```python
from build123d import *
from build123d import SkipClean  # not in build123d's __all__

# Parameters (mm, degrees)
F1_DEPTH = 31.75
F3_DEPTH = 12.7
F5_DEPTH = 12.7
F7_DEPTH = 25.401


with BuildPart() as f1:
    # F0 (on Top) → F1 (new body)
    with BuildSketch(Plane.XY):
        Polygon((31.597598396, 0), (0, -0.0003033445), (0, -38.1), (31.75, -38.1), (31.75, -25.4), (57.15, -25.4), (57.15, -12.7), (31.597598396, -12.7), align=None)
    extrude(amount=F1_DEPTH)

    # F2 (on face) → F3 (cut)
    with BuildSketch(Plane.XZ.offset(38.1)):
        Polygon((31.75, 0), (31.75, 31.75), (19.05, 31.75), align=None)
    extrude(amount=-F3_DEPTH, mode=Mode.SUBTRACT)

    # F4 (on face) → F5 (cut)
    with BuildSketch(Plane(origin=(2.9e-09, -0.0003033445, 0), x_dir=(-1, -9.6002e-06, 0), z_dir=(-9.6002e-06, 1, 0))):
        Polygon((-18.8975983945, 31.75), (-31.5975983945, 31.75), (-31.5975983945, 0), align=None)
    with SkipClean():  # cleaning this boolean's faces spoils the solid; the shape is the same uncleaned
        extrude(amount=-F5_DEPTH, mode=Mode.SUBTRACT)

    # F6 (on face) → F7 (cut, through all)
    with BuildSketch(Plane(origin=(0, -12.7, 0), x_dir=(-1, 0, 0), z_dir=(0, 1, 0))):
        Polygon((-44.373799198, 31.75), (-57.15, 31.75), (-57.15, 0), align=None)
    extrude(amount=-F7_DEPTH, mode=Mode.SUBTRACT)


solid = f1.part
```
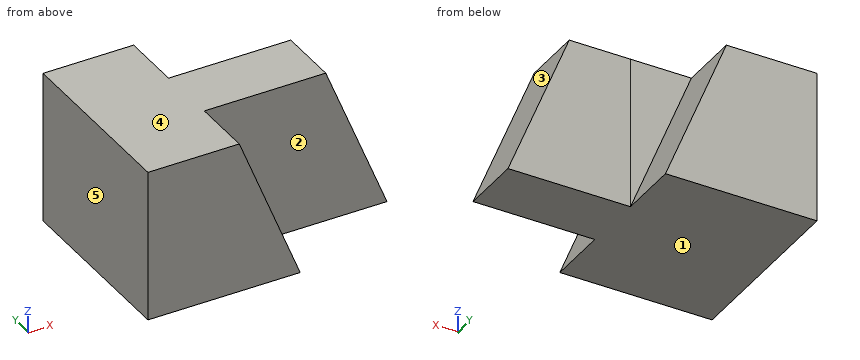
Design review of the part built by this model. Coordinates are the model's own, in mm. Face numbers are marked on the shaded views. A direction names the side the tool comes from. Give positions to 0.01 mm unless a question says otherwise; leave off trailing zeros. Order: outer loops, then holes, each group sorted by start corner. A loop starts at its lowest first (then second) coordinate and runs counter-clockwise, first axis right, second up. Notation, with made-up numbers: (44.25, -15) -> (85.25, -15) arc R26 ccw to (85.25, 4) -> close; hole circle Ø8 at (39, 61). An arc over 180 degrees is marked (long way). Write item = value, one per line. Start each with the question number.
(1) Mouldability with a two-part tool opening along X and no side actions: class the marked faces 3, 4 and 5 as +X half, -X half, draft (parallel to the pull), parting line (faces both ways), or undercut.
(2) We need section A-A on x = 23. Write out the cut boundary in (y, z) (3 decimals).
(3) For the marked faces 1 and 2, list the 3-axis set-ups (+Z, -Z, +X, -X, +Y, -Y) from which the entire face can be reached by the end or side of a thin tool; tool diameter is ignored.
(4) We need section D-D on z = 15. Write out the cut boundary in (x, y), plus the area to 3 significant figures.
(5) For pin 1 (2 mm diameter, centred on x = 19, y = -5, fed in from +Z); pin 2 (2 mm diameter, centred on x = 32, z = 9, fed in from -Y); pin 3 (1.5 mm diameter, centred on y = -4, z = 8, fed in from +X), all flat-tipped, find the tip position at first contact; note any pin that passes through.
(6) We need section B-B on z = 22. Write out the cut boundary in (x, y), plus the area to 3 significant figures.
(7) To check wall thickness, follow line 1 along Y through (x, z) = (47.5, 2.5); line 2 along X through (y, z) = (-15, 22.5); line 3 along X through (y, z) = (-7, 17). State the ranges of each line that lie inside material, in increasing order.
Numbers:
q1.face_3 = +X half
q1.face_4 = draft
q1.face_5 = -X half
q2.outline = (-38.1, 0) -> (0, 0) -> (0, 21.494) -> (-12.7, 21.494) -> (-12.7, 31.75) -> (-25.4, 31.75) -> (-25.4, 21.875) -> (-38.1, 21.875) -> close
q3.face_1 = -Z, +X, -X, +Y, -Y
q3.face_2 = +Z, +X, -Y
q4.outline = (0, -38.1) -> (25.75, -38.1) -> (25.75, -25.4) -> (51.11, -25.4) -> (51.11, -12.7) -> (31.6, -12.7) -> (25.6, -12.7) -> (25.6, 0) -> (0, 0) -> close
q4.area = 1,300 mm^2
q5.pin_1 = 31.75
q5.pin_2 = -25.4
q5.pin_3 = 28.7
q6.outline = (0, -38.1) -> (22.95, -38.1) -> (22.95, -25.4) -> (48.3, -25.4) -> (48.3, -12.7) -> (31.6, -12.7) -> (22.8, -12.7) -> (22.8, 0) -> (0, 0) -> close
q6.area = 1,190 mm^2
q7.line_1 = -25.4 to -12.7
q7.line_2 = 0 to 48.1
q7.line_3 = 0 to 24.8
